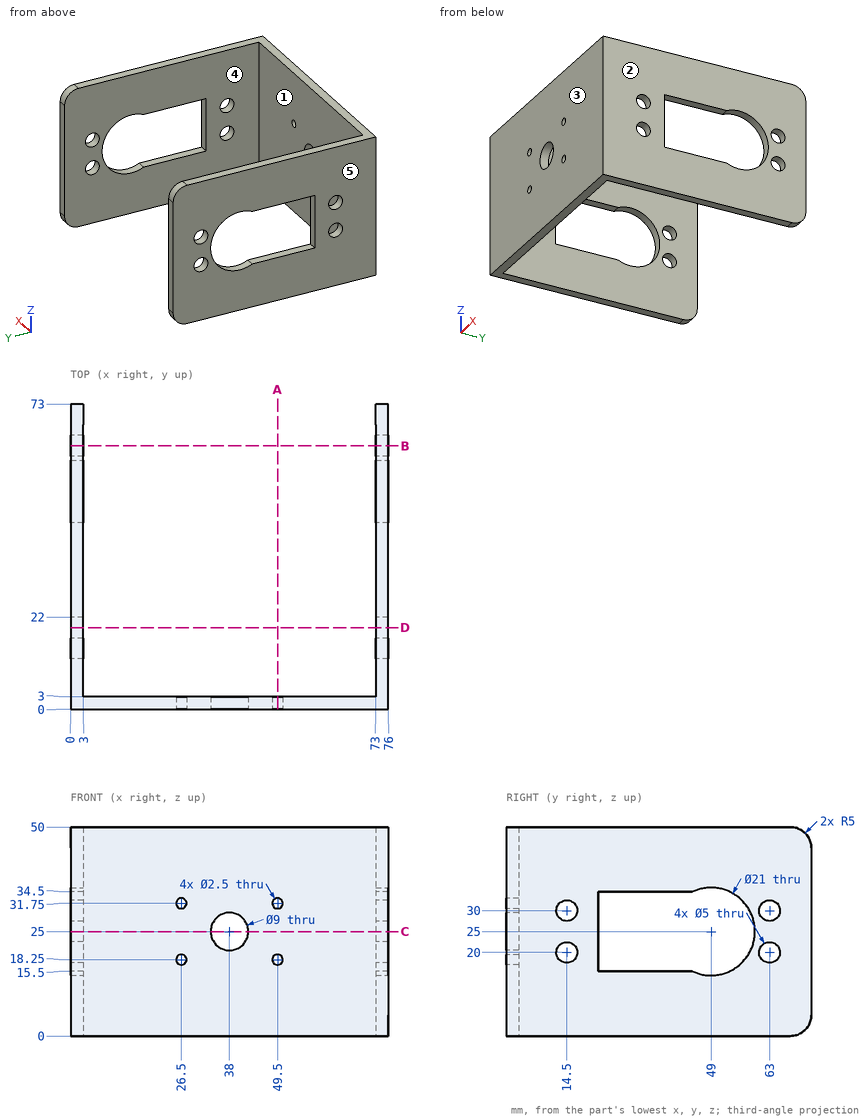
Answer from the drawing. Dimensions are ordinates in mm from the lowest x, y and z of the part. A direction names the side the tool comes from. Give positions to 0.01 mm unless a question says otherwise; leave off trailing zeros. Write each loop counter-clockwise with the first axis right and the second up, starting at its lowest first coordinate (ties: lowest second). Pieces come first, ordered by that corner, then holes. Notation, with made-up numbers: (-33.5, 75) - (12.5, 75) arc R29 ccw to (12.5, 109) - close; hole circle Ø6 at (37.25, -3.75). An arc over 180 degrees is marked (long way). Answer in a Markdown table with one row per item. Add a question column.
Item 1: Flat-ended cylindrical pins translate along their axes: P1, Ø4, axis at x = 49.5, z = 31.75, coming from the +Y side; P2, Ø4.5, axis at y = 14.5, z = 20, coming from the +X side. Find the tip coordinate at first contact, or state that the pin passes through.
Item 2: Section B-B, the plane y = 63 is taken. Write down the section's boundary in (x, z).
Item 3: Find the intervals of material crossed by L1, parallel to Z at x = 74.7, y = 14.5; L2, parallel to Z at x = 1.05, y = 49; L3, parallel to Y at x = 74.45, z = 25, in increasing order.
Item 4: Determine the mould class of the marked faces 1, 2 and 3 for opening direction X: pulls with the +X half, pulls with the -X half, needs draft (parallel to the pull), parting line crosses it, or undercut.
Item 5: Section D-D, the plane y = 19.5 is taken. Write down the section's boundary in (x, z), and give its area (3 significant figures).
Item 6: Section C-C, the plane z = 25 is taken. Write down the section's boundary in (x, y).
Item 7: Section A-A, the plane x = 49.5 is taken. Write down the section's boundary in (y, z).
Item 8: A tool of negligible diameter and unlimited length cuts with its end or side. For the marked faces 4 and 5, from which of +Z, -Z, +X, -X, +Y, -Y can it reach the whole face along a straight path? Write none if from no direction.
Recorded:
| question | item | result |
|---|---|---|
| 1 | P1 | stops at y = 3 |
| 1 | P2 | passes through |
| 2 | outline | (0, 0) - (3, 0) - (3, 17.5) - (0, 17.5) - close; (0, 22.5) - (3, 22.5) - (3, 27.5) - (0, 27.5) - close; (0, 32.5) - (3, 32.5) - (3, 50) - (0, 50) - close; (73, 0) - (76, 0) - (76, 17.5) - (73, 17.5) - close; (73, 22.5) - (76, 22.5) - (76, 27.5) - (73, 27.5) - close; (73, 32.5) - (76, 32.5) - (76, 50) - (73, 50) - close |
| 3 | L1 | z = 0 to 17.5, 22.5 to 27.5, 32.5 to 50 |
| 3 | L2 | z = 0 to 14.5, 35.5 to 50 |
| 3 | L3 | y = 0 to 22, 59.5 to 73 |
| 4 | face 1 | undercut |
| 4 | face 2 | pulls with the +X half |
| 4 | face 3 | needs draft |
| 5 | outline | (0, 0) - (3, 0) - (3, 50) - (0, 50) - close; (73, 0) - (76, 0) - (76, 50) - (73, 50) - close |
| 5 | area | 300 mm2 |
| 6 | outline | (0, 0) - (33.5, 0) - (33.5, 3) - (3, 3) - (3, 22) - (0, 22) - close; (0, 59.5) - (3, 59.5) - (3, 73) - (0, 73) - close; (42.5, 0) - (76, 0) - (76, 22) - (73, 22) - (73, 3) - (42.5, 3) - close; (73, 59.5) - (76, 59.5) - (76, 73) - (73, 73) - close |
| 7 | outline | (0, 0) - (3, 0) - (3, 17) - (0, 17) - close; (0, 19.5) - (3, 19.5) - (3, 30.5) - (0, 30.5) - close; (0, 33) - (3, 33) - (3, 50) - (0, 50) - close |
| 8 | face 4 | +Z, -Z, +Y |
| 8 | face 5 | +Z, -Z, -X, +Y, -Y |
